The model under review builds one solid part; all positions refer to its coordinate system, in mm. A direction names the side the tool comes from. Coordinates: 2 decimals unless noted, no trailing zeros. Write each loop counter-clockwise with the first axis right and the second up, starting at its lowest first coordinate (ties: lowest second). Pieces come first, ordered by that corner, then holes.
```python
from build123d import *

# Parameters (mm, degrees)
SKETCH1_W           = 200
SKETCH1_H           = 40
BOSS_EXTRUDE1_DEPTH = 2.7
SKETCH2_R           = 1.75
CUT_EXTRUDE1_DEPTH  = 3.7
SKETCH3_R           = 1.75
CUT_EXTRUDE2_DEPTH  = 3.7
SKETCH4_R           = 1.75
CUT_EXTRUDE3_DEPTH  = 3.7
SKETCH5_R           = 1.75
CUT_EXTRUDE4_DEPTH  = 3.7
LPATTERN2_COUNT     = 2
LPATTERN2_PITCH     = 9.5
SKETCH6_R           = 1.75
CUT_EXTRUDE5_DEPTH  = 3.7
SKETCH7_R           = 1.75
CUT_EXTRUDE6_DEPTH  = 3.7
SKETCH8_R           = 2.5
CUT_EXTRUDE7_DEPTH  = 3.7
LPATTERN3_COUNT     = 9
LPATTERN3_PITCH     = 22.5
BOSS_EXTRUDE2_DEPTH = 200


with BuildPart() as part:
    # Sketch1 → Boss-Extrude1 (new body)
    with BuildSketch(Plane(origin=(0, 0, 0), x_dir=(1, 0, 0), z_dir=(0, 1, 0))):
        Rectangle(SKETCH1_W, SKETCH1_H)
    extrude(amount=BOSS_EXTRUDE1_DEPTH)

    # Sketch2 → Cut-Extrude1 (cut, through all)
    with BuildSketch(Plane(origin=(0, 2.7, 0), x_dir=(1, 0, 0), z_dir=(0, 1, 0))):
        with Locations((-90.2, 15)):
            Circle(SKETCH2_R)
    extrude(amount=-CUT_EXTRUDE1_DEPTH, mode=Mode.SUBTRACT)

    # Sketch3 → Cut-Extrude2 (cut, through all)
    with BuildSketch(Plane(origin=(0, 2.7, 0), x_dir=(1, 0, 0), z_dir=(0, 1, 0))):
        with Locations((-77.2, 15)):
            Circle(SKETCH3_R)
    extrude(amount=-CUT_EXTRUDE2_DEPTH, mode=Mode.SUBTRACT)

    # Sketch4 → Cut-Extrude3 (cut, through all)
    with BuildSketch(Plane(origin=(0, 2.7, 0), x_dir=(1, 0, 0), z_dir=(0, 1, 0))):
        with Locations((-67.7, 15)):
            Circle(SKETCH4_R)
    extrude(amount=-CUT_EXTRUDE3_DEPTH, mode=Mode.SUBTRACT)

    # Sketch5 → Cut-Extrude4 (cut, through all)
    with BuildSketch(Plane(origin=(0, 2.7, 0), x_dir=(1, 0, 0), z_dir=(0, 1, 0))):
        with Locations((-54.7, 15)):
            Circle(SKETCH5_R)
    cut_extrude4 = extrude(amount=-CUT_EXTRUDE4_DEPTH, mode=Mode.SUBTRACT)

    # LPattern2: Cut-Extrude4 ×2
    with Locations(*[(i * LPATTERN2_PITCH, 0, 0) for i in range(1, LPATTERN2_COUNT)]):
        add(cut_extrude4, mode=Mode.SUBTRACT)

    # Sketch6 → Cut-Extrude5 (cut, through all)
    with BuildSketch(Plane(origin=(0, 2.7, 0), x_dir=(1, 0, 0), z_dir=(0, 1, 0))):
        with Locations((-32.2, 15)):
            Circle(SKETCH6_R)
        with Locations((-22.7, 15)):
            Circle(SKETCH6_R)
    extrude(amount=-CUT_EXTRUDE5_DEPTH, mode=Mode.SUBTRACT)

    # Sketch7 → Cut-Extrude6 (cut, through all)
    with BuildSketch(Plane(origin=(0, 2.7, 0), x_dir=(1, 0, 0), z_dir=(0, 1, 0))):
        with Locations((-9.7, 15)):
            Circle(SKETCH7_R)
        with Locations((-0.2, 15)):
            Circle(SKETCH7_R)
        with Locations((12.8, 15)):
            Circle(SKETCH7_R)
        with Locations((22.3, 15)):
            Circle(SKETCH7_R)
        with Locations((35.3, 15)):
            Circle(SKETCH7_R)
        with Locations((44.8, 15)):
            Circle(SKETCH7_R)
        with Locations((57.8, 15)):
            Circle(SKETCH7_R)
        with Locations((67.3, 15)):
            Circle(SKETCH7_R)
        with Locations((80.3, 15)):
            Circle(SKETCH7_R)
        with Locations((89.8, 15)):
            Circle(SKETCH7_R)
    extrude(amount=-CUT_EXTRUDE6_DEPTH, mode=Mode.SUBTRACT)

    # Sketch8 → Cut-Extrude7 (cut, through all)
    with BuildSketch(Plane(origin=(0, 2.7, 0), x_dir=(1, 0, 0), z_dir=(0, 1, 0))):
        with Locations((-95, -15)):
            Circle(SKETCH8_R)
    cut_extrude7 = extrude(amount=-CUT_EXTRUDE7_DEPTH, mode=Mode.SUBTRACT)

    # LPattern3: Cut-Extrude7 ×9
    with Locations(*[(i * LPATTERN3_PITCH, 0, 0) for i in range(1, LPATTERN3_COUNT)]):
        add(cut_extrude7, mode=Mode.SUBTRACT)

    # Sketch10 → Boss-Extrude2 (add)
    with BuildSketch(Plane(origin=(100, 0, 0), x_dir=(0, 0, -1), z_dir=(1, 0, 0))):
        Polygon((-10, 0), (-10, -20), (5, 0), align=None)
    extrude(amount=-BOSS_EXTRUDE2_DEPTH)


solid = part.part
```
Item 1: Take a section at A-A, the plane x = -90.2. Write out the cut boundary in (y, z).
Solved:
outline: (-20, 10) - (0, -5) - (0, -13.25) - (2.7, -13.25) - (2.7, 20) - (0, 20) - (0, 10) - close; (0, -20) - (2.7, -20) - (2.7, -16.75) - (0, -16.75) - close
Item 2: Take a section at D-D, the plane y = -17. Write out the cut boundary in (x, z).
Solved:
outline: (-100, 7.75) - (100, 7.75) - (100, 10) - (-100, 10) - close
Item 3: Take a section at C-C, the plane z = -15. Count the separate pieces of the cut face and the enclosed holes in it, plus the area to 3 significant figures.
Solved:
separate pieces: 18
enclosed holes: 0
area: 379 mm2
Item 4: For pin 1 (4 mm diameter, centred on x = -35, y = -9, fed in from +Z); pin 2 (3 mm diameter, centred on x = 67.3, z = -15, fed in from +Y); pin 3 (3 mm diameter, centred on x = -42, z = 15, fed in from -Y); pin 4 (12 mm diameter, centred on x = -4, z = -9, fed in from -Y), all flat-tipped, find the tip position at first contact; note any pin that passes through.
Solved:
pin 1: stops at z = 10
pin 2: passes through
pin 3: stops at y = 0
pin 4: stops at y = -2.67
Item 5: Mouldability with a two-part tool opening along X and no side actions: class faces 1 (the face through (1, -10, 10)), 2 (the face through (100, -4, 3)), 3 (the face through (-29, 1, 17)) as pulls with the +X half, pulls with the -X half, needs draft (parallel to the pull), parting line crosses it, or undercut.
Solved:
face 1: needs draft
face 2: pulls with the +X half
face 3: undercut
Item 6: Take a section at B-B, the plane x = 3.5. Write out the cut boundary in (y, z).
Solved:
outline: (-20, 10) - (0, -5) - (0, -20) - (2.7, -20) - (2.7, 20) - (0, 20) - (0, 10) - close
Item 7: Machinability: for faces 4 (the face through (-1, 0, 15)), 5 (the face through (-97, 1.4, 16.5)), 6 (the face through (-1, 0, -13)), which of the approach directions +Z, -Z, +X, -X, +Y, -Y give a long, thin tool a straight path to every point of the face, cutting with its end or side? Answer none if there is none.
Solved:
face 4: +Z, +X, -X, -Y
face 5: +Y, -Y
face 6: -Z, +X, -X, -Y
Item 8: To check wall thickness, follow line 1 along Z through (x, y) = (35.5, 0.5); line 2 along Z through (x, y) = (-72.5, 1.75); line 3 along Y through (x, z) = (-6, -5). State the ranges of each line that lie inside material, in increasing order.
Solved:
line 1: z = -20 to -16.74, -13.26 to 20
line 2: z = -20 to 12.5, 17.5 to 20
line 3: y = 0 to 2.7
